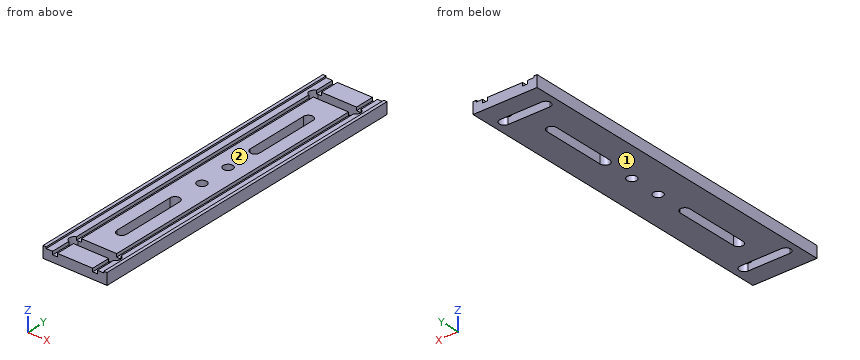
```python
from build123d import *

# Parameters (mm, degrees)
F0_W     = 20
F0_H     = 105
F1_DEPTH = 3.1
F2_W     = 1
F2_H     = 105
F3_DEPTH = 0.5
F4_R     = 1.5
F5_DEPTH = 3.101
F6_W     = 1.5
F6_H     = 105
F7_DEPTH = 1


with BuildPart() as f1:
    # F0 (on Top) → F1 (new body)
    with BuildSketch(Plane.XY):
        with Locations((10, 52.5)):
            Rectangle(F0_W, F0_H)
    extrude(amount=F1_DEPTH)

    # F2 (on face) → F3 (join)
    with BuildSketch(Plane.XY.offset(3.1)):
        with Locations((19.5, 52.5)):
            Rectangle(F2_W, F2_H)
        with Locations((0.5, 52.5)):
            Rectangle(F2_W, F2_H)
    extrude(amount=F3_DEPTH)

    # F4 (on face) → F5 (cut, through all)
    with BuildSketch(Plane.XY.offset(3.1)):
        with BuildLine():
            Line((16.5, 9), (3.5, 9))
            ThreePointArc((3.5, 9), (2, 7.5), (3.5, 6))
            Line((3.5, 6), (16.5, 6))
            ThreePointArc((16.5, 6), (18, 7.5), (16.5, 9))
        make_face()
        with BuildLine():
            Line((8.5, 37.5), (8.5, 17.5))
            ThreePointArc((8.5, 17.5), (10, 16), (11.5, 17.5))
            Line((11.5, 17.5), (11.5, 37.5))
            ThreePointArc((11.5, 37.5), (10, 39), (8.5, 37.5))
        make_face()
        with Locations((10, 47.6)):
            Circle(F4_R)
        with BuildLine():
            Line((16.5, 99), (3.5, 99))
            ThreePointArc((3.5, 99), (2, 97.5), (3.5, 96))
            Line((3.5, 96), (16.5, 96))
            ThreePointArc((16.5, 96), (18, 97.5), (16.5, 99))
        make_face()
        with BuildLine():
            Line((11.5, 67.5), (11.5, 87.5))
            ThreePointArc((11.5, 87.5), (10, 89), (8.5, 87.5))
            Line((8.5, 87.5), (8.5, 67.5))
            ThreePointArc((8.5, 67.5), (10, 66), (11.5, 67.5))
        make_face()
        with Locations((10, 57.4)):
            Circle(F4_R)
    extrude(amount=-F5_DEPTH, mode=Mode.SUBTRACT)

    # F6 (on face) → F7 (cut)
    with BuildSketch(Plane.XY.offset(3.1)):
        with Locations((3.75, 52.5)):
            Rectangle(F6_W, F6_H)
        with Locations((16.25, 52.5)):
            Rectangle(F6_W, F6_H)
    extrude(amount=-F7_DEPTH, mode=Mode.SUBTRACT)


solid = f1.part
```
Geometry: final body of the model. Coordinates: model frame, mm. Face numbers are marked on the shaded views. A direction names the side the tool comes from. Coordinates: 2 decimals unless noted, no trailing zeros. Order: outer loops, then holes, each group sorted by start corner. A loop starts at its lowest first (then second) coordinate and runs counter-clockwise, first axis right, second up. Notation, with made-up numbers: M 14.25,82.25 L 18.25,82.25 A23 cw 18.25,96.25 Z; hole C 56.5,-35 d8. An arc over 180 degrees is marked long. Answer as CSV lines item,"result".
Q1. Section C-C on z = 0.9. Return the cut outline in (x, y), and give its area (3 significant figures).
Answers:
outline,"M 0,0 L 20,0 L 20,105 L 0,105 Z; hole M 3.5,6 L 16.5,6 A1.5 ccw 16.5,9 L 3.5,9 A1.5 ccw Z; hole M 3.5,96 L 16.5,96 A1.5 ccw 16.5,99 L 3.5,99 A1.5 ccw Z; hole M 8.5,17.5 A1.5 ccw 11.5,17.5 L 11.5,37.5 A1.5 ccw 8.5,37.5 Z; hole C 10,47.6 d3; hole C 10,57.4 d3; hole M 8.5,67.5 A1.5 ccw 11.5,67.5 L 11.5,87.5 A1.5 ccw 8.5,87.5 Z"
area,"1,860 mm^2"
Q2. Set-up query: the marked faces 1 and 2. Return all of +Z, -Z, +X, -X, +Y, -Y with unobstructed straight access to the full face (end or side cutting, diameter ignored); none if empty.
Answers:
face 1,"-Z, +X, -X, +Y, -Y"
face 2,"+Z, +Y, -Y"
Q3. Section D-D on x = 9.5. Return the cut outline in (y, z), and give its area (3 significant figures).
Answers:
outline,"M 0,0 L 6,0 L 6,3.1 L 0,3.1 Z; M 9,0 L 16.09,0 L 16.09,3.1 L 9,3.1 Z; M 38.91,0 L 46.19,0 L 46.19,3.1 L 38.91,3.1 Z; M 49.01,0 L 55.99,0 L 55.99,3.1 L 49.01,3.1 Z; M 58.81,0 L 66.09,0 L 66.09,3.1 L 58.81,3.1 Z; M 88.91,0 L 96,0 L 96,3.1 L 88.91,3.1 Z; M 99,0 L 105,0 L 105,3.1 L 99,3.1 Z"
area,"148 mm^2"
Q4. First-contact query: P1, Ø6, axis at x = 4.5, y = 60, coming from the +Z side; P2, Ø2.5, axis at x = 10, y = 57.4, coming from the -Z side; P3, Ø0.8, axis at x = 4, y = 4, coming from the +Z side. Flat tips, straight axial feed; report the tip coordinate or a pass-through.
Answers:
P1,"stops at z = 3.1"
P2,"passes through"
P3,"stops at z = 2.1"
Q5. Line query: probe 1 along X at (y, z) = (12, 2.45); probe 2 along Y at (x, z) = (12.5, 2.35); probe 3 along X at (y, z) = (74, 2.8). Output: solid intervals per line, ascending. Write a range as [from, to].
Answers:
probe 1,"x = [0, 3], [4.5, 15.5], [17, 20]"
probe 2,"y = [0, 6], [9, 96], [99, 105]"
probe 3,"x = [0, 3], [4.5, 8.5], [11.5, 15.5], [17, 20]"
Q6. Section B-B on y = 47.6. Return the cut outline in (x, z).
Answers:
outline,"M 0,0 L 8.5,0 L 8.5,3.1 L 4.5,3.1 L 4.5,2.1 L 3,2.1 L 3,3.1 L 1,3.1 L 1,3.6 L 0,3.6 Z; M 11.5,0 L 20,0 L 20,3.6 L 19,3.6 L 19,3.1 L 17,3.1 L 17,2.1 L 15.5,2.1 L 15.5,3.1 L 11.5,3.1 Z"
Q7. Section A-A on x = 14.5. Return the cut outline in (y, z).
Answers:
outline,"M 0,0 L 6,0 L 6,3.1 L 0,3.1 Z; M 9,0 L 96,0 L 96,3.1 L 9,3.1 Z; M 99,0 L 105,0 L 105,3.1 L 99,3.1 Z"
